from build123d import *

# Parameters (mm, degrees)
SKETCH1_W               = 8
SKETCH1_H               = 8
BOSS_EXTRUDE1_DEPTH     = 3
CUT_EXTRUDE1_DEPTH      = 12.704699911
CUT_EXTRUDE1_DEPTH_BACK = 12.704699911
CUT_EXTRUDE2_DEPTH      = 11
SKETCH4_R               = 1.8
CUT_EXTRUDE3_DEPTH      = 0.8
SKETCH5_W               = 8
SKETCH5_H               = 1
BOSS_EXTRUDE2_DEPTH     = 2
FILLET1_R               = 4
CUT_EXTRUDE4_DEPTH      = 0.4


with BuildPart() as part:
    # Sketch1 → Boss-Extrude1 (new body)
    with BuildSketch(Plane(origin=(0, 0, 0), x_dir=(1, 0, 0), z_dir=(0, 1, 0))):
        with Locations((4, 4)):
            Rectangle(SKETCH1_W, SKETCH1_H)
    extrude(amount=BOSS_EXTRUDE1_DEPTH)

    # Sketch2 → Cut-Extrude1 (cut, two sides: drawn at the far end of the back side and taken through both)
    with BuildSketch(Plane.XY.offset(-CUT_EXTRUDE1_DEPTH_BACK)):
        Polygon((0, 0), (0.6, 3), (0, 3), align=None)
        Polygon((8, 0), (7.4, 3), (8, 3), align=None)
    extrude(amount=CUT_EXTRUDE1_DEPTH + CUT_EXTRUDE1_DEPTH_BACK, mode=Mode.SUBTRACT)

    # Sketch3 → Cut-Extrude2 (cut)
    with BuildSketch(Plane(origin=(0, 0, 0), x_dir=(0, 0, -1), z_dir=(1, 0, 0))):
        Polygon((0, 0), (0.6, 3), (0, 3), align=None)
        Polygon((8, 3), (7.4, 3), (8, 0), align=None)
    extrude(amount=CUT_EXTRUDE2_DEPTH, mode=Mode.SUBTRACT)

    # Sketch4 → Cut-Extrude3 (cut)
    with BuildSketch(Plane.XZ):
        with Locations(Location((4, -3.75, 0), (0, 0, 270))):
            Circle(SKETCH4_R)
    extrude(amount=-CUT_EXTRUDE3_DEPTH, mode=Mode.SUBTRACT)

    # Sketch5 → Boss-Extrude2 (add)
    with BuildSketch(Plane.XZ):
        with Locations((4, -7.5)):
            Rectangle(SKETCH5_W, SKETCH5_H)
    extrude(amount=BOSS_EXTRUDE2_DEPTH)

    # Fillet1
    # the kernel refuses this fillet: 4 mm, written as the material it takes off along each edge
    with BuildSketch(Plane(origin=(8, -2, -16.660254038), x_dir=(0, 1, 0), z_dir=(0, 0, 1)), Plane(origin=(0, -2, 1.660254038), x_dir=(0, 1, 0), z_dir=(0, 0, -1))) as fillet1_piece_1:
        with BuildLine():
            CenterArc((4, 3.464101615), FILLET1_R, 180, 60)
            Line((0, 3.464101615), (-0.08, 3.464101615))
            Line((-0.08, 3.464101615), (-0.08, 0))
            Line((-0.08, 0), (0, -0.08))
            ThreePointArc((0, -0.08), (1, -0.08), (1.96, -0.069282032))
            Line((1.96, -0.069282032), (2, 0))
        make_face()
    extrude(amount=18.320508076, mode=Mode.SUBTRACT)

    # Sketch6 → Cut-Extrude4 (cut)
    with BuildSketch(Plane(origin=(0, 3, 0), x_dir=(1, 0, 0), z_dir=(0, 1, 0))):
        with BuildLine():
            Line((4.053794593, 3.505457585), (4.053794593, 4.172124252))
            Line((4.053794593, 4.172124252), (5.797384337, 4.172124252))
            Line((5.797384337, 4.172124252), (5.797384337, 2.564752457))
            add(Edge.make_bspline(
                [(5.797384337, 2.564752457), (5.775440275, 2.544992361), (5.730582172, 2.504598726), (5.657391115, 2.447633596), (5.576814656, 2.393249062), (5.489339896, 2.340343698), (5.394785806, 2.289343315), (5.293529517, 2.239537607), (5.185384208, 2.19141366), (5.032450931, 2.131128575), (4.835594452, 2.065533422), (4.594933471, 2.008496304), (4.352368706, 1.973513189), (4.190125473, 1.969167013), (4.109083055, 1.966996047)],
                knots=[0, 0, 0, 0, 0.581799769, 1.189316438, 1.825828404, 2.496525428, 3.203088405, 3.942228803, 4.719818701, 5.534979611, 7.181138583, 8.803804008, 10.403462225, 12, 12, 12, 12], degree=3))
            add(Edge.make_bspline(
                [(4.109083055, 1.966996047), (4.058312627, 1.967758979), (3.958229013, 1.969262944), (3.810482794, 1.981368296), (3.667847904, 2.002080495), (3.530208107, 2.031409962), (3.397097502, 2.066765974), (3.26907094, 2.111868039), (3.146582956, 2.166009466), (3.028523806, 2.226338905), (2.917094396, 2.295632176), (2.812187083, 2.371432832), (2.714561168, 2.454400196), (2.624566637, 2.544701507), (2.540998329, 2.641714843), (2.464831298, 2.745902822), (2.396526155, 2.857385727), (2.335239765, 2.974765127), (2.280716867, 3.097008702), (2.234709094, 3.223154334), (2.194374003, 3.351370526), (2.161222966, 3.482107416), (2.136875151, 3.615790052), (2.117947657, 3.751799892), (2.107781758, 3.890986734), (2.105984472, 3.984609884), (2.105076645, 4.031899893)],
                knots=[0, 0, 0, 0, 1.124918047, 2.217548049, 3.282233239, 4.316494221, 5.334437038, 6.332151046, 7.320712088, 8.300141923, 9.267552434, 10.225301062, 11.165776911, 12.103230934, 13.047553934, 14.000517593, 14.959782875, 15.941944936, 16.932894943, 17.923491392, 18.915624898, 19.910402922, 20.909870877, 21.92519501, 22.95199481, 24, 24, 24, 24], degree=3))
            add(Edge.make_bspline(
                [(2.105076645, 4.031899893), (2.105812881, 4.082940857), (2.107264322, 4.183564655), (2.119773705, 4.33228546), (2.139199297, 4.476648194), (2.168656936, 4.616390773), (2.20449512, 4.75216369), (2.248233589, 4.883877531), (2.301822866, 5.010556427), (2.361436063, 5.133283761), (2.429297714, 5.250362339), (2.505977563, 5.360290437), (2.589206445, 5.464176802), (2.680629029, 5.560371285), (2.779923369, 5.648827012), (2.886080088, 5.730522243), (2.998844963, 5.806865303), (3.079553832, 5.849911113), (3.120301004, 5.871643482)],
                knots=[0, 0, 0, 0, 1.105010302, 2.178452875, 3.229459892, 4.257086284, 5.268538906, 6.268935615, 7.259234261, 8.24469117, 9.221745683, 10.185929258, 11.144249683, 12.101504986, 13.055838221, 14.020611351, 15.000673771, 16, 16, 16, 16], degree=3))
            add(Edge.make_bspline(
                [(3.120301004, 5.871643482), (3.152638085, 5.887700047), (3.218317351, 5.920312247), (3.322813337, 5.959248923), (3.432101667, 5.994677516), (3.547832356, 6.021111591), (3.6692195, 6.042829226), (3.796209305, 6.059036287), (3.929210312, 6.067547239), (4.019595582, 6.068879104), (4.065813824, 6.069560149)],
                knots=[0, 0, 0, 0, 0.887969848, 1.803539625, 2.741143579, 3.713741423, 4.722068772, 5.775476617, 6.8624965, 8, 8, 8, 8], degree=3))
            add(Edge.make_bspline(
                [(4.065813824, 6.069560149), (4.125403824, 6.06867255), (4.241295356, 6.066946335), (4.410256532, 6.05256252), (4.569271079, 6.027772487), (4.718560435, 5.993629866), (4.857802985, 5.949731518), (4.986759025, 5.895763799), (5.106220057, 5.832812796), (5.214455834, 5.758355608), (5.313666102, 5.676257846), (5.403591975, 5.586419647), (5.48426965, 5.488707943), (5.555752499, 5.383614392), (5.617477906, 5.2707046), (5.670549966, 5.151008328), (5.714234697, 5.023616882), (5.73534656, 4.935145779), (5.746102286, 4.89007297)],
                knots=[0, 0, 0, 0, 1.271135529, 2.472123572, 3.614091059, 4.701890498, 5.736279567, 6.724681829, 7.680621489, 8.611506429, 9.52200816, 10.424540711, 11.318996785, 12.221421405, 13.131851814, 14.060431888, 15.011860567, 16, 16, 16, 16], degree=3))
            Line((5.746102286, 4.89007297), (4.976871517, 4.736226816))
            add(Edge.make_bspline(
                [(4.976871517, 4.736226816), (4.969254672, 4.761468809), (4.95422678, 4.81127079), (4.925094227, 4.882758251), (4.891539922, 4.949961192), (4.853483379, 5.013366036), (4.810541206, 5.072582433), (4.761675926, 5.126971617), (4.709961453, 5.179014495), (4.652020351, 5.225088646), (4.590259767, 5.266624284), (4.52537561, 5.304078684), (4.455901775, 5.334453158), (4.382811411, 5.358892727), (4.306461756, 5.37964837), (4.225856415, 5.392413169), (4.141900573, 5.402040295), (4.084540473, 5.402606041), (4.055397158, 5.402893482)],
                knots=[0, 0, 0, 0, 1.027736275, 2.027704492, 3.005900071, 3.954421694, 4.908588141, 5.853155543, 6.803277083, 7.766271258, 8.734041521, 9.704274878, 10.683578894, 11.68490234, 12.708089448, 13.76461009, 14.864251086, 16, 16, 16, 16], degree=3))
            add(Edge.make_bspline(
                [(4.055397158, 5.402893482), (4.01128773, 5.401716629), (3.925204424, 5.399419898), (3.799534269, 5.384433236), (3.680976007, 5.357770589), (3.569219615, 5.320994553), (3.46406021, 5.273789934), (3.366918824, 5.2143961), (3.275376693, 5.146327474), (3.192038786, 5.066438045), (3.116460773, 4.976859168), (3.051034483, 4.876522357), (2.996567377, 4.765751945), (2.951955713, 4.645104141), (2.91643531, 4.514573915), (2.892338718, 4.373699188), (2.876594443, 4.222696077), (2.875085403, 4.118480819), (2.874307414, 4.064752457)],
                knots=[0, 0, 0, 0, 1.043810997, 2.037086103, 2.989314757, 3.91471467, 4.817033861, 5.710208705, 6.603920097, 7.511448416, 8.435617211, 9.371747005, 10.338444094, 11.350425613, 12.411431869, 13.5347293, 14.729025275, 16, 16, 16, 16], degree=3))
            add(Edge.make_bspline(
                [(2.874307414, 4.064752457), (2.875118698, 4.00702506), (2.876695474, 3.894828493), (2.892027057, 3.732262921), (2.917247643, 3.580803592), (2.95342224, 3.44064155), (2.998941149, 3.311279521), (3.053656914, 3.192304252), (3.121182779, 3.085923464), (3.197244894, 2.990004781), (3.28225913, 2.906191636), (3.37384152, 2.833121051), (3.471482188, 2.77119638), (3.576081527, 2.721395085), (3.686320303, 2.681751972), (3.80321198, 2.653959398), (3.926408504, 2.636695674), (4.010734238, 2.634687946), (4.053794593, 2.633662713)],
                knots=[0, 0, 0, 0, 1.318042826, 2.561693173, 3.724929596, 4.821196409, 5.862977565, 6.853497791, 7.804600806, 8.73339865, 9.643480846, 10.524649628, 11.404635349, 12.277659519, 13.165160235, 14.075017549, 15.017020959, 16, 16, 16, 16], degree=3))
            add(Edge.make_bspline(
                [(4.053794593, 2.633662713), (4.097408334, 2.634875039), (4.185053042, 2.637311287), (4.316328539, 2.657956024), (4.448117665, 2.68833542), (4.577327471, 2.734163302), (4.70281192, 2.786727561), (4.819965055, 2.847306941), (4.929675356, 2.910453005), (4.995733738, 2.959668979), (5.028153568, 2.98382297)],
                knots=[0, 0, 0, 0, 0.993821502, 1.997150276, 3.023717651, 4.073291794, 5.118404464, 6.123376694, 7.078999408, 8, 8, 8, 8], degree=3))
            Line((5.028153568, 2.98382297), (5.028153568, 3.505457585))
            Line((5.028153568, 3.505457585), (4.053794593, 3.505457585))
        make_face()
    extrude(amount=-CUT_EXTRUDE4_DEPTH, mode=Mode.SUBTRACT)


solid = part.part
Input: part model. Units: mm. Frame: model coordinates. A direction names the side the tool comes from. Coordinates: 2 decimals unless noted, no trailing zeros. Order: outer loops, then holes, each group sorted by start corner. A loop starts at its lowest first (then second) coordinate and runs counter-clockwise, first axis right, second up. Notation, with made-up numbers: M -6,18.5 L 35,18.5 A31 ccw 35,49.5 Z; hole C 71.5,60 d6. An arc over 180 degrees is marked long. Answer in a Markdown table with one row per item.
(1) Draft query along Z for faces 1 (the flat face through (4.4, 2.6, -4)), 2 (the flat face through (4, -1, -8)), 3 (the flat face through (4, 0.8, -4)), 4 (the flat face through (3, 0, -2)). Return one class per face: pulls with the +Z half, pulls with the -Z half, needs draft (parallel to the pull), parting line crosses it, or undercut.
Numbers:
| item | result |
|---|---|
| face 1 | undercut |
| face 2 | pulls with the -Z half |
| face 3 | undercut |
| face 4 | needs draft |
(2) Material intervals for line 1 (Y direction, x = 5.5, z = -5); line 2 (Y direction, x = 3, z = -6); line 3 (X direction, y = 2.8, z = -4), sorted ascending. Write a range as [from, to].
Numbers:
| item | result |
|---|---|
| line 1 | y = [0, 2.6] |
| line 2 | y = [0, 3] |
| line 3 | x = [0.56, 2.11], [2.88, 4.05], [5.8, 7.44] |
(3) Contact query for flat-ended pins moving along their axis: pin 1 Ø1 at (y, z) = (-1, -5) entering from -X; pin 2 Ø3 at (x, z) = (4, -3.75) entering from -Y; pin 3 Ø3 at (x, y) = (6, 2) entering from +Z; pin 4 Ø1 at (y, z) = (2, -1) entering from +X. Output: stop coordinate, or through.
Numbers:
| item | result |
|---|---|
| pin 1 | passes through |
| pin 2 | stops at y = 0.8 |
| pin 3 | stops at z = -0.1 |
| pin 4 | stops at x = 7.7 |
(4) Section query B-B, the plane x = 1.5. Output: boundary loops of the cut face in (y, z).
Numbers:
| item | result |
|---|---|
| outline | M -1.48,-8 L 0,-8 L 3,-7.4 L 3,-0.6 L 0,0 L 0,-7 L -1.48,-7 Z |
(5) Access query for faces 5 (the cylindrical face through (4.541, 0.394, -5.467)), 6 (the flat face through (4, -1, -7)), 7 (the cylindrical face through (1.49, -1.48, -7.49)). Directions: +Z, -Z, +X, -X, +Y, -Y. A direction counts if a zero-diameter tool reaches every point of the face in a straight line with its end or side. Return the directions, or none.
Numbers:
| item | result |
|---|---|
| face 5 | -Y |
| face 6 | +Z, +X, -X, -Y |
| face 7 | +Z, -Z, -X, -Y |
(6) Section query D-D, the plane z = -6.25. Output: boundary loops of the cut face in (x, y).
Numbers:
| item | result |
|---|---|
| outline | M 0,0 L 8,0 L 7.4,3 L 0.6,3 Z |
(7) Section query A-A, the plane y = 0.35. Output: boundary loops of the cut face in (x, z), plus the area to 3 significant figures.
Numbers:
| item | result |
|---|---|
| outline | M 0.07,-7.93 L 7.93,-7.93 L 7.93,-0.07 L 0.07,-0.07 Z; hole C 4,-3.75 d3.6 |
| area | 51.6 mm^2 |
(8) Section query C-C, the plane y = 2. Output: boundary loops of the cut face in (x, z), plus the area to 3 significant figures.
Numbers:
| item | result |
|---|---|
| outline | M 0.4,-7.6 L 7.6,-7.6 L 7.6,-0.4 L 0.4,-0.4 Z |
| area | 51.8 mm^2 |
